Part model, mm, in its own coordinate system. Face numbers are marked on the shaded views. Give positions to 0.01 mm unless a question says otherwise; leave off trailing zeros. Order: outer loops, then holes, each group sorted by start corner. A loop starts at its lowest first (then second) coordinate and runs counter-clockwise, first axis right, second up. Notation, with made-up numbers: (-28.5, -27) - (12.5, -27) arc R6 cw to (12.5, -18) - close; hole circle Ø5 at (-39.5, 18.25). An arc over 180 degrees is marked (long way). One line per item, written item: value.
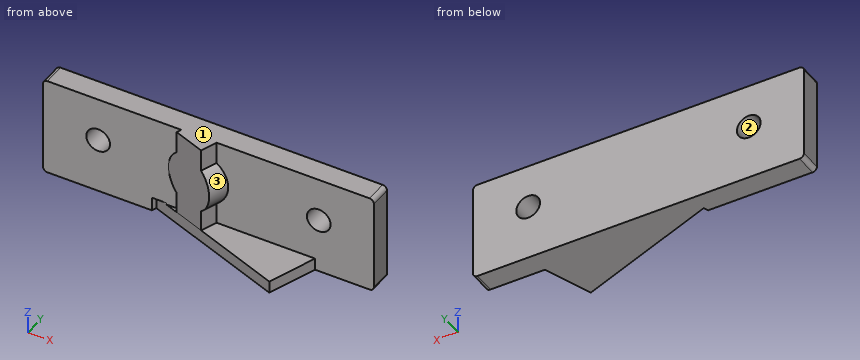
```python
from build123d import *

# Parameters (mm, degrees)
SKETCH_1_W          = 60
SKETCH_1_H          = 18
SKETCH_1_R          = 2.15
EXTRUDE_1_DEPTH     = 4
EXTRUDE_3_DEPTH     = 2.2
CUT_EXTRUDE_1_DEPTH = 2.5
EXTRUDE_2_DEPTH     = 3.981010851
FILLET_1_R          = 0.8


with BuildPart() as part:
    # 草图1 → 凸台-拉伸1 (new body)
    with BuildSketch(Plane(origin=(0, 0, 0), x_dir=(1, 0, 0), z_dir=(0, 1, 0))):
        with Locations((0, 9)):
            Rectangle(SKETCH_1_W, SKETCH_1_H)
        with Locations(Location((-20, 8, 0), (0, 0, 270))):
            Circle(SKETCH_1_R, mode=Mode.SUBTRACT)
        with Locations(Location((20, 8, 0), (0, 0, 270))):
            Circle(SKETCH_1_R, mode=Mode.SUBTRACT)
    extrude(amount=EXTRUDE_1_DEPTH)

    # 草图5 → 凸台-拉伸3 (add)
    with BuildSketch(Plane(origin=(0, 0, -18), x_dir=(-1, 0, 0), z_dir=(0, 0, -1))):
        Polygon((-19.332346445, 0), (10.038960076, 0), (10.380980219, -0.939692621), (-15.554536115, -10.379448577), align=None)
    extrude(amount=-EXTRUDE_3_DEPTH)

    # 草图6 → 切除-拉伸1 (cut)
    with BuildSketch(Plane(origin=(0, 0, -18), x_dir=(-1, 0, 0), z_dir=(0, 0, -1))):
        Polygon((-16.365155241, -8.73705171), (-9.866772518, -26.591211505), (16.444620864, -17.014647492), (9.946238141, 0.839512303), align=None)
    extrude(amount=-CUT_EXTRUDE_1_DEPTH, mode=Mode.SUBTRACT)

    # 草图4 → 凸台-拉伸2 (add)
    with BuildSketch(Plane(origin=(0.467911114, 1.285575219, 0), x_dir=(0, 0, -1), z_dir=(0.34202014332566943, 0.9396926207859081, 0))):
        with BuildLine():
            Line((0, 4.633536704), (4, 4.633536704))
            ThreePointArc((4, 4.633536704), (8, 6.633536704), (12, 4.633536704))
            Line((12, 4.633536704), (18, 4.633536704))
            Line((18, 4.633536704), (18, -1.366463296))
            Line((18, -1.366463296), (12, -1.366463296))
            ThreePointArc((12, -1.366463296), (8, -3.366463296), (4, -1.366463296))
            Line((4, -1.366463296), (0, -1.366463296))
            Line((0, -1.366463296), (0, 4.633536704))
        make_face()
    extrude(amount=-EXTRUDE_2_DEPTH)

    # 圆角1
    fillet_1_edges = [part.edges().sort_by_distance(p)[0] for p in [
        (-30, 2, -18),
        (30, 2, -18),
        (30, 2, 0),
        (-30, 2, 0),
    ]]
    fillet(fillet_1_edges, radius=FILLET_1_R)


solid = part.part
```
1) Slice it at D-D on x = 14.5. Write the cut outline in (y, z).
Answer:
outline: (-8.06, -18) - (4, -18) - (4, 0) - (0, 0) - (0, -15.8) - (-8.06, -15.8) - close
2) Slice it at B-B on z = -7. Write the cut outline in (x, y).
Answer:
outline: (-30, 0) - (-21.9, 0) - (-21.9, 4) - (-30, 4) - close; (-18.1, 0) - (-6.95, 0) - (-7.03, -0.22) - (2.17, -3.57) - (3.48, 0) - (18.1, 0) - (18.1, 4) - (-18.1, 4) - close; (21.9, 0) - (30, 0) - (30, 4) - (21.9, 4) - close
3) Slice it at A-A on x = -20. Write the cut outline in (y, z), then the cut area to 3 significant figures.
Answer:
outline: (0, -18) - (4, -18) - (4, -10.15) - (0, -10.15) - close; (0, -5.85) - (4, -5.85) - (4, 0) - (0, 0) - close
area: 54.8 mm2
4) Slice it at C-C on z = -3. Write the cut outline in (x, y), then the cut area to 3 significant figures.
Answer:
outline: (-30, 0) - (-4.93, 0) - (-5.25, -0.87) - (0.39, -2.92) - (1.45, 0) - (30, 0) - (30, 4) - (-30, 4) - close
area: 252 mm2
5) Two-plate mould, pull along X, no slides. Class the marked faces 1, 2 and 3: pulls with the +X half, pulls with the -X half, needs draft (parallel to the pull), parting line crosses it, or undercut.
Answer:
face 1: needs draft
face 2: undercut
face 3: pulls with the +X half
6) Drop flat-ended pins along their axis: P1, Ø2, axis at x = 15.5, y = -4.5, coming from the +Z side; P2, Ø4, axis at x = -17, z = -13, coming from the -Y side; P3, Ø2, axis at y = -2.5, z = -10, coming from the +X side; P4, Ø2.5, axis at x = 20, z = -8, coming from the +Y side. Give the stop position or say it passes through.
Answer:
P1: stops at z = -15.8
P2: stops at y = 0
P3: stops at x = 2.75
P4: passes through
7) Wall check: line 1 along X through (y, z) = (1.35, -8); line 2 along Y through (x, z) = (19, -12.5); line 3 along X through (y, z) = (2.5, -6.5). Give the ranges that are in metal, low to high. Write a range as [from, to].
Answer:
line 1: x = [-30, -22.15], [-17.85, 17.85], [22.15, 30]
line 2: y = [0, 4]
line 3: x = [-30, -21.54], [-18.46, 18.46], [21.54, 30]
